Read the model definition and answer for the solid it produces. Units are mm, in the model's axes. A direction names the side the tool comes from. Round coordinates to 2 decimals unless told otherwise and drop trailing zeros. Order: outer loops, then holes, each group sorted by start corner. A loop starts at its lowest first (then second) coordinate and runs counter-clockwise, first axis right, second up. Notation, with made-up numbers: (-33, 45.25) - (-2, 45.25) arc R16 cw to (-2, 70.25) - close; hole circle Ø6 at (9.25, 13). An arc over 180 degrees is marked (long way). Answer as a JSON object with one key per item and string values. Group by question number.
Q1. A cutting plane is placed at A-A on z = 33.5. Determine the outline of the cut face in (x, y), and give its area (3 significant figures).
Q2. Given pin 1 Ø4 at (x, z) = (15, 50) entering from +Y; pin 2 Ø6 at (y, z) = (-5.5, 7.5) entering from -X; pin 3 Ø1.2 at (x, z) = (-15, 18.5) entering from -Y, each flat-ended and moving along its own axis, determine where each tip first touches the part or whether it passes through.
Q3. Consider line 1 (X direction, y = 4.25, z = 0.5); line 2 (Z direction, x = -8.5, y = -2.75); line 3 (Y direction, x = 15, z = 15). Determine where each line is inside the solid, lowest interval first.
Q4. A cutting plane is placed at D-D on x = 7. Determine the outline of the cut face in (y, z), and give its area (3 significant figures).
Q5. A tool of negligible diameter and unlimited length cuts with its end or side. For faces 1 (the flat face through (14.3, 0, 30)), 2 (the flat face through (-16, -5, 30)), 3 (the flat face through (-15, 5, 30)), from which of +Z, -Z, +X, -X, +Y, -Y can it reach the whole face along a straight path? Write none if from no direction.
Q6. A cutting plane is placed at B-B on x = -16. Determine the outline of the cut face in (y, z), and give its area (3 significant figures).
Q7. The mould has two halves that part along X. Classify faces 4 (the flat face through (-19, 0, -5)), 5 (the flat face through (0, 0, -10)), 6 (the flat face through (19, 0, -5)), 7 (the flat face through (-14.3, 0, 30)): pulls with the +X half, pulls with the -X half, needs draft (parallel to the pull), parting line crosses it, or undercut.
Q8. A cutting plane is placed at C-C on y = 1.25. Determine the outline of the cut face in (x, z), and give its area (3 significant figures).
```python
from build123d import *

# Parameters (mm, degrees)
F2_DEPTH = 60
F1_W     = 38
F1_H     = 15
F3_DEPTH = 10


with BuildPart() as f2:
    # F0 (on Top) → F2 (new body)
    with BuildSketch(Plane.XY):
        Polygon((14.3, 5), (14.3, 0), (14.3, -5), (16.7, -5), (16.7, 5), align=None)
    extrude(amount=F2_DEPTH)



with BuildPart() as f2b:
    # F0 (on Top) → F2, piece 2 (new body)
    with BuildSketch(Plane.XY):
        Polygon((-14.3, -5), (-14.3, 0), (-14.3, 5), (-16.7, 5), (-16.7, -5), align=None)
    extrude(amount=F2_DEPTH)


with BuildPart() as f2_1:
    add(f2.part)

    add(f2b.part)  # F3 merges F2b
    # F1 (on Top) → F3 (join)
    with BuildSketch(Plane.XY):
        Rectangle(F1_W, F1_H)
    extrude(amount=-F3_DEPTH)


solid = f2_1.part
```
Result set:
{
 "1": {"outline": "(-16.7, -5) - (-14.3, -5) - (-14.3, 5) - (-16.7, 5) - close; (14.3, -5) - (16.7, -5) - (16.7, 5) - (14.3, 5) - close", "area": "48.0 mm²"},
 "2": {"pin 1": "stops at y = 5", "pin 2": "stops at x = -16.7", "pin 3": "stops at y = -5"},
 "3": {"line 1": "x = -16.7 to -14.3, 14.3 to 16.7", "line 2": "z = -10 to 0", "line 3": "y = -5 to 5"},
 "4": {"outline": "(-7.5, -10) - (7.5, -10) - (7.5, 0) - (-7.5, 0) - close", "area": "150 mm²"},
 "5": {"face 1": "+Z, +Y, -Y", "face 2": "+Z, +X, -X, -Y", "face 3": "+Z, +X, -X, +Y"},
 "6": {"outline": "(-7.5, -10) - (7.5, -10) - (7.5, 0) - (5, 0) - (5, 60) - (-5, 60) - (-5, 0) - (-7.5, 0) - close", "area": "750 mm²"},
 "7": {"face 4": "pulls with the -X half", "face 5": "needs draft", "face 6": "pulls with the +X half", "face 7": "undercut"},
 "8": {"outline": "(-19, -10) - (19, -10) - (19, 0) - (16.7, 0) - (16.7, 60) - (14.3, 60) - (14.3, 0) - (-14.3, 0) - (-14.3, 60) - (-16.7, 60) - (-16.7, 0) - (-19, 0) - close", "area": "668 mm²"}
}
